Check sheet for the drawn part. Datum: minimum x, y, z corner. Units: mm. A direction names the side the tool comes from. Coordinates: 2 decimals unless noted, no trailing zeros. Order: outer loops, then holes, each group sorted by start corner. A loop starts at its lowest first (then second) coordinate and runs counter-clockwise, first axis right, second up. Notation, with made-up numbers: (83.25, 27.25) - (117.25, 27.25) arc R23 ccw to (117.25, 38.25) - close; hole circle Ø7 at (-19.5, 10.25). An arc over 180 degrees is marked (long way). Return JSON: item names as keys, results as strings. Group by question number.
Item 1: Gauge pin test, flat ends, axial feed: pin 1 (0.8 mm diameter, centred on x = 6, z = 1.5, fed in from -Y); pin 2 (3 mm diameter, centred on x = 7, z = 2.5, fed in from -Y); pin 3 (2 mm diameter, centred on x = 5.5, z = 3, fed in from +Y). Record the tip position at first contact, or that the pin passes through.
Item 2: Tool access check on the marked faces 5, 6 and 7. Record the directions out of +Z, -Z, +X, -X, +Y, -Y that give a thin tool (end or side, any length) a straight path to the whole face; none if there is none.
Item 3: Scan lines: probe 1 along Y at (x, z) = (6.25, 2.65); probe 2 along X at (y, z) = (13, 2.25); probe 3 along X at (y, z) = (12.5, 2.95). Record each from-to range of solid material in increasing order.
Item 4: Draft check along X on the marked faces 1, 2, 3 and 4. Enter one of: pulls with the +X half, pulls with the -X half, needs draft (parallel to the pull), parting line crosses it, or undercut.
Item 5: Section check A-A on x = 5.5. Enter the section's corners in (y, z), then the cut area to 3 significant figures.
Item 6: Section check B-B on z = 2.1. Enter the section's corners in (x, y), then the cut area to 3 significant figures.
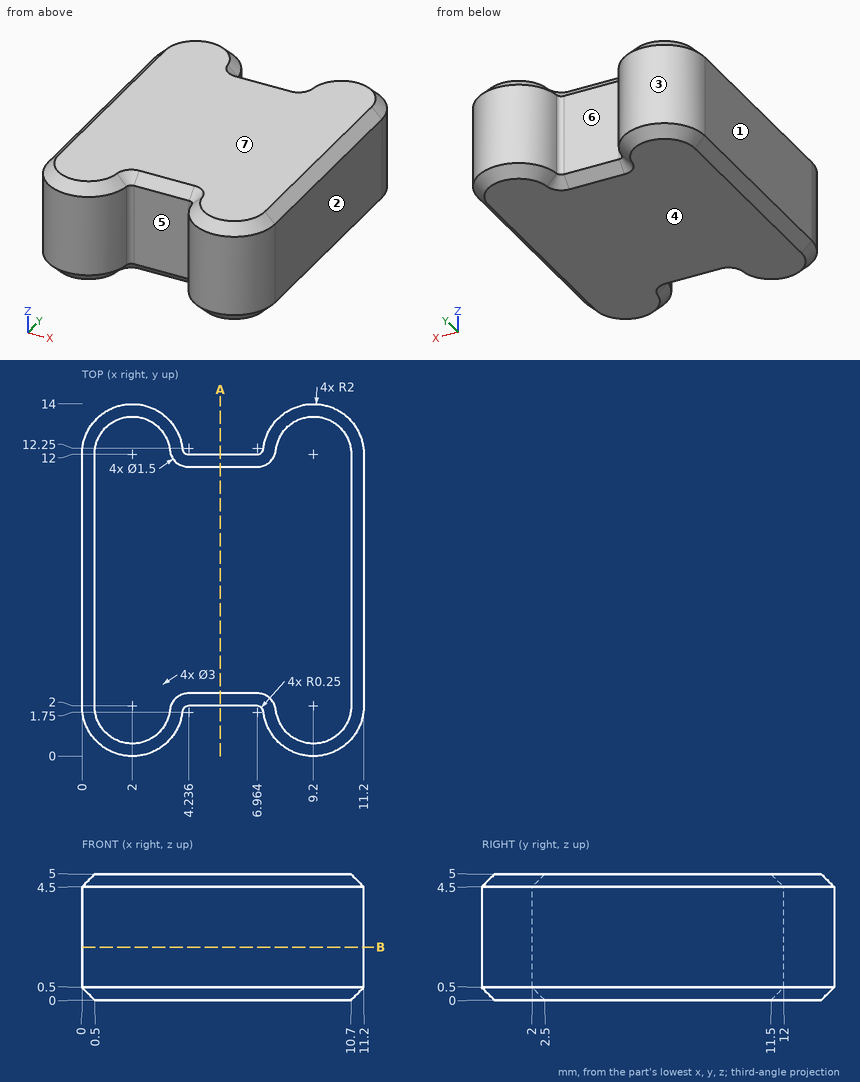
Computed:
{
 "1": {"pin 1": "stops at y = 2", "pin 2": "stops at y = 0.13", "pin 3": "stops at y = 12"},
 "2": {"face 5": "+Z, -Z, -Y", "face 6": "+Z, -Z, +Y", "face 7": "+Z, +X, -X, +Y, -Y"},
 "3": {"probe 1": "y = 2 to 12", "probe 2": "x = 0.27 to 3.73, 7.47 to 10.93", "probe 3": "x = 0.06 to 3.94, 7.26 to 11.14"},
 "4": {"face 1": "pulls with the -X half", "face 2": "pulls with the +X half", "face 3": "undercut", "face 4": "needs draft"},
 "5": {"outline": "(2, 0.5) - (2.5, 0) - (11.5, 0) - (12, 0.5) - (12, 4.5) - (11.5, 5) - (2.5, 5) - (2, 4.5) - close", "area": "49.5 mm²"},
 "6": {"outline": "(0, 2) arc R2 ccw to (3.99, 1.78) arc R0.25 cw to (4.24, 2) - (6.96, 2) arc R0.25 cw to (7.21, 1.78) arc R2 ccw to (11.2, 2) - (11.2, 12) arc R2 ccw to (7.21, 12.22) arc R0.25 cw to (6.96, 12) - (4.24, 12) arc R0.25 cw to (3.99, 12.22) arc R2 ccw to (0, 12) - close", "area": "137 mm²"}
}
